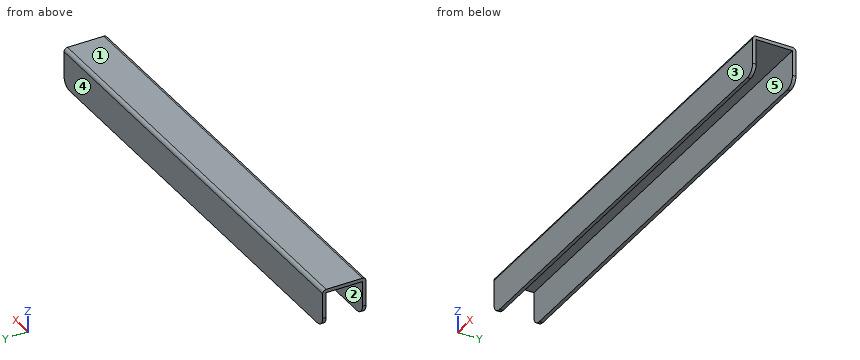
from build123d import *

# Parameters (mm, degrees)
F0_W     = 298.45
F0_H     = 28.575
F1_DEPTH = 2.286
F2_W     = 298.45
F2_H     = 2.286
F3_DEPTH = 23.114
F4_R     = 2.286
F5_R     = 6.35
F6_R     = 6.35
F7_R     = 6.35


with BuildPart() as f1:
    # F0 (on Top) → F1 (new body)
    with BuildSketch(Plane.XY):
        Rectangle(F0_W, F0_H)
    extrude(amount=F1_DEPTH)

    # F2 (on face) → F3 (join)
    with BuildSketch(Plane(origin=(0, 0, 0), x_dir=(1, 0, 0), z_dir=(0, 0, -1))):
        with Locations((0, 13.1445)):
            Rectangle(F2_W, F2_H)
        with Locations((0, -13.1445)):
            Rectangle(F2_W, F2_H)
    extrude(amount=F3_DEPTH)

    # F4
    f4_edges = [f1.edges().sort_by_distance(p)[0] for p in [
        (0, -14.2875, 2.286),
        (0, 14.2875, 2.286),
    ]]
    fillet(f4_edges, radius=F4_R)

    # F5
    f5_edges = [f1.edges().sort_by_distance(p)[0] for p in [
        (149.225, -13.1445, -23.114),
    ]]
    fillet(f5_edges, radius=F5_R)

    # F6
    f6_edges = [f1.edges().sort_by_distance(p)[0] for p in [
        (149.225, 13.1445, -23.114),
    ]]
    fillet(f6_edges, radius=F6_R)

    # F7
    f7_edges = [f1.edges().sort_by_distance(p)[0] for p in [
        (-149.225, -13.1445, -23.114),
        (-149.225, 13.1445, -23.114),
    ]]
    fillet(f7_edges, radius=F7_R)


solid = f1.part
Design review of the part built by this model. Coordinates are the model's own, in mm. Face numbers are marked on the shaded views. A direction names the side the tool comes from. Coordinates: 2 decimals unless noted, no trailing zeros. Order: outer loops, then holes, each group sorted by start corner. A loop starts at its lowest first (then second) coordinate and runs counter-clockwise, first axis right, second up. Notation, with made-up numbers: M -38,61 L 9,61 A12 cw 9,67 Z; hole C 13.5,21 d8. An arc over 180 degrees is marked long. Use a Markdown table: item, result.
(1) Wall thickness on probe 1 along Y at (x, z) = (-7, -21.75); probe 2 along Z at (x, y) = (0, 3); probe 3 along Y at (x, z) = (-51.5, 0.75): over which ranges is each line inside the solid? List them lowest first.
Worked answers:
| item | result |
|---|---|
| probe 1 | y = -14.29 to -12, 12 to 14.29 |
| probe 2 | z = 0 to 2.29 |
| probe 3 | y = -14.16 to 14.16 |
(2) For P1, Ø6, axis at x = 103, y = 7.5, coming from the -Z side; P2, Ø10, axis at y = -7.5, z = -13, coming from the +X side (3 decimals), all flat-tipped, find the tip position at first contact; note any pin that passes through.
Worked answers:
| item | result |
|---|---|
| P1 | stops at z = 0 |
| P2 | stops at x = 149.225 |
(3) Add section C-C (y = -8.5). Give the boundary of the cut face in (x, z) (3 decimals), then the cut area to 3 significant figures.
Worked answers:
| item | result |
|---|---|
| outline | M -149.225,0 L 149.225,0 L 149.225,2.286 L -149.225,2.286 Z |
| area | 682 mm2 |
(4) For the marked faces 4 and 5, list the 3-axis set-ups (+Z, -Z, +X, -X, +Y, -Y) from which the entire face can be reached by the end or side of a thin tool; tool diameter is ignored.
Worked answers:
| item | result |
|---|---|
| face 4 | +Z, -Z, +X, -X, +Y |
| face 5 | -Z, +X, -X |
(5) Draft analysis for pull direction Y (two halves, no side actions). For the marked faces 1, 2 and 3, state which applies: released by +Y, released by -Y, zero draft, split by the parting line, or undercut.
Worked answers:
| item | result |
|---|---|
| face 1 | zero draft |
| face 2 | undercut |
| face 3 | released by -Y |
(6) Add section A-A (z = -13). Give the boundary of the cut face in (x, y) (1 decimal).
Worked answers:
| item | result |
|---|---|
| outline | M -149.2,-14.3 L 149.2,-14.3 L 149.2,-12 L -149.2,-12 Z; M -149.2,12 L 149.2,12 L 149.2,14.3 L -149.2,14.3 Z |
(7) Add section B-B (x = 119.5). Give the boundary of the cut face in (y, z), then the cut area to 3 significant figures.
Worked answers:
| item | result |
|---|---|
| outline | M -14.29,-23.11 L -12,-23.11 L -12,0 L 12,0 L 12,-23.11 L 14.29,-23.11 L 14.29,0 A2.29 ccw 12,2.29 L -12,2.29 A2.29 ccw -14.29,0 Z |
| area | 169 mm2 |
